Read the model definition and answer for the solid it produces. Units are mm, in the model's axes. A direction names the side the tool comes from. Coordinates: 2 decimals unless noted, no trailing zeros. Loops run counter-clockwise (first coordinate to the right, second up) from the corner with the lowest first, then second, coordinate; pieces in that order, holes last.
Q1. Straight lines are drawn through the part: line 1 (Z direction, x = 0, y = -0.7); line 2 (Y direction, x = 44, z = 29); line 3 (X direction, y = -20, z = -6). For each, find the intervals that lie inside material, in ascending order.
Q2. Flat-ended cylindrical pins translate along their axes: P1, Ø6, axis at x = 40.5, y = -11.5, coming from the -Z side; P2, Ø1, axis at y = -21, z = 14, coming from the +X side; P3, Ø16, axis at x = 0, z = 0, coming from the +Y side; P4, Ø22, axis at x = 1.5, z = -0.5, coming from the -Y side. Find the tip coordinate at first contact, or state that the pin passes through.
Q3. The mould has two halves that part along X. Classify faces 4 (the face through (-33, 0, 48)), 5 (the face through (-26.76, -0.49, -51.46)), 6 (the face through (-24.268, -31.209, 1.068)): pulls with the +X half, pulls with the -X half, needs draft (parallel to the pull), parting line crosses it, or undercut.
Q4. Which of the six approach directions +Z, -Z, +X, -X, +Y, -Y give full straight-line access (tool end or side, diameter ignored) to faces 1 (the face through (24, -25.5, -24)), 2 (the face through (-13.87, -8.63, -62.48)), 3 (the face through (1, -1, 1))?
Q5. Section B-B (y = -29) is taken. Give the vertices of the cut face in (x, z), then the cut area to 3 significant figures.
Q6. Section D-D (y = -3.5) is taken. Give the vertices of the cut face in (x, z).
from build123d import *

# Parameters (mm, degrees)
F0_R      = 64
F1_DEPTH  = 25.5
F2_R      = 58
F3_DEPTH  = 1
F4_SIZE   = 8
F5_R      = 30
F6_DEPTH  = 6
F7_SIZE   = 5.99999
F9_R      = 10
F10_DEPTH = 18


# Not quite as in the source:
# - a fillet or chamfer is up to 0.001 mm smaller than in the source, because OpenCascade refuses the exact size


with BuildPart() as f1:
    # F0 (on Front) → F1 (new body)
    with BuildSketch(Plane.XZ):
        Circle(F0_R)
    extrude(amount=F1_DEPTH)

    # F2 (on face) → F3 (cut)
    with BuildSketch(Plane(origin=(0, 0, 0), x_dir=(-1, 0, 0), z_dir=(0, 1, 0))):
        Circle(F2_R)
    extrude(amount=-F3_DEPTH, mode=Mode.SUBTRACT)

    # F4
    f4_edges = [f1.edges().sort_by_distance(p)[0] for p in [
        (-64, -25.5, 0),
    ]]
    chamfer(f4_edges, length=F4_SIZE)

    # F5 (on face) → F6 (join)
    with BuildSketch(Plane.XZ.offset(25.5)):
        Circle(F5_R)
    extrude(amount=F6_DEPTH)

    # F7 (size 6 in the source; OpenCascade refuses exactly that, so slightly less here)
    f7_edges = [f1.edges().sort_by_distance(p)[0] for p in [
        (-30, -31.5, 0),
    ]]
    chamfer(f7_edges, length=F7_SIZE)

    # F9 (on face) → F10 (cut)
    with BuildSketch(Plane.XZ.offset(31.5)):
        Circle(F9_R)
    extrude(amount=-F10_DEPTH, mode=Mode.SUBTRACT)


solid = f1.part
Numbers:
1. line 1: z = -64 to -58, 58 to 64
1. line 2: y = -25.5 to -1
1. line 3: x = -61.21 to -8, 8 to 61.21
2. P1: stops at z = -51.86
2. P2: stops at x = 59.38
2. P3: stops at y = -1
2. P4: stops at y = -31.5
3. face 4: needs draft
3. face 5: undercut
3. face 6: parting line crosses it
4. face 1: -Y
4. face 2: +Y, -Y
4. face 3: +Y
5. outline: circle Ø53 at (0, 0); hole circle Ø20 at (0, 0)
5. area: 1,890 mm2
6. outline: circle Ø128 at (0, 0)
